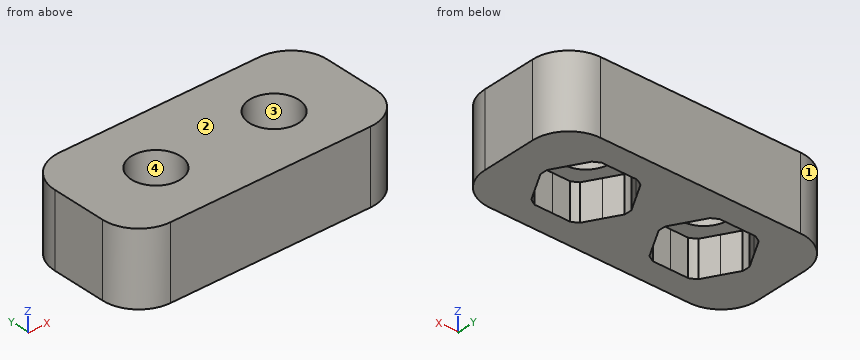
Solid Edge part; units mm, degrees
sketch "Sketch1" plane through (0, 0, 0) normal (0, 0, 1) x (1, 0, 0)
  line L0 (-4.5, -7) -> (17.5, -7)
  arc A0 (17.5, -7) -> (21.5, -3) centre (17.5, -3) ccw
  line L1 (21.5, -3) -> (21.5, 3)
  arc A1 (21.5, 3) -> (17.5, 7) centre (17.5, 3) ccw
  line L2 (17.5, 7) -> (-4.5, 7)
  arc A2 (-4.5, 7) -> (-8.5, 3) centre (-4.5, 3) ccw
  line L3 (-8.5, 3) -> (-8.5, -3)
  arc A3 (-8.5, -3) -> (-4.5, -7) centre (-4.5, -3) ccw
extrude "Protrusion1" add sketch "Sketch1" along normal blind 8
sketch "Sketch2" plane through (0, 0, 0) normal (0, 0, 1) x (1, 0, 0)
  line L0 (-1.9421, -4.225) -> (0, -4.225)
  line L1 (1.9421, -4.225) -> (0, -4.225)
  arc A0 (2.6879, -3.7944) -> (1.9421, -4.225) centre (0, 0) cw
  line L2 (2.6879, -3.7944) -> (3.659, -2.1125)
  line L3 (4.63, -0.4306) -> (3.659, -2.1125)
  arc A1 (4.63, 0.4306) -> (4.63, -0.4306) centre (0, 0) cw
  line L4 (4.63, 0.4306) -> (3.659, 2.1125)
  line L5 (2.6879, 3.7944) -> (3.659, 2.1125)
  arc A2 (1.9421, 4.225) -> (2.6879, 3.7944) centre (0, 0) cw
  line L6 (1.9421, 4.225) -> (0, 4.225)
  line L7 (-1.9421, 4.225) -> (0, 4.225)
  arc A3 (-2.6879, 3.7944) -> (-1.9421, 4.225) centre (0, 0) cw
  line L8 (-2.6879, 3.7944) -> (-3.659, 2.1125)
  line L9 (-4.63, 0.4306) -> (-3.659, 2.1125)
  arc A4 (-4.63, -0.4306) -> (-4.63, 0.4306) centre (0, 0) cw
  line L10 (-4.63, -0.4306) -> (-3.659, -2.1125)
  line L11 (-2.6879, -3.7944) -> (-3.659, -2.1125)
  arc A5 (-1.9421, -4.225) -> (-2.6879, -3.7944) centre (0, 0) cw
  line L12 (11.0579, -4.225) -> (13, -4.225)
  line L13 (14.9421, -4.225) -> (13, -4.225)
  arc A6 (15.6879, -3.7944) -> (14.9421, -4.225) centre (13, 0) cw
  line L14 (15.6879, -3.7944) -> (16.659, -2.1125)
  line L15 (17.63, -0.4306) -> (16.659, -2.1125)
  arc A7 (17.63, 0.4306) -> (17.63, -0.4306) centre (13, 0) cw
  line L16 (17.63, 0.4306) -> (16.659, 2.1125)
  line L17 (15.6879, 3.7944) -> (16.659, 2.1125)
  arc A8 (14.9421, 4.225) -> (15.6879, 3.7944) centre (13, 0) cw
  line L18 (14.9421, 4.225) -> (13, 4.225)
  line L19 (11.0579, 4.225) -> (13, 4.225)
  arc A9 (10.3121, 3.7944) -> (11.0579, 4.225) centre (13, 0) cw
  line L20 (10.3121, 3.7944) -> (9.341, 2.1125)
  line L21 (8.37, 0.4306) -> (9.341, 2.1125)
  arc A10 (8.37, -0.4306) -> (8.37, 0.4306) centre (13, 0) cw
  line L22 (8.37, -0.4306) -> (9.341, -2.1125)
  line L23 (10.3121, -3.7944) -> (9.341, -2.1125)
  arc A11 (11.0579, -4.225) -> (10.3121, -3.7944) centre (13, 0) cw
extrude "ExtrudedCutout_1" cut sketch "Sketch2" along normal blind 4
sketch "Sketch3" plane through (0, 0, 0) normal (0, 0, 1) x (1, 0, 0)
  circle A0 centre (0, 0) radius 2.7
  circle A1 centre (13, 0) radius 2.7
extrude "Cutout1" cut sketch "Sketch3" along normal through all
chamfer "Chamfer_1" [suppressed]
properties material "ABS Plastic, medium impact"
Input: part model. Units: mm. Frame: model coordinates. Face numbers are marked on the shaded views. Coordinates: 2 decimals unless noted, no trailing zeros. Loops run counter-clockwise (first coordinate to the right, second up) from the corner with the lowest first, then second, coordinate; pieces in that order, holes last. Notation, with made-up numbers: M 48,58 L 89,58 A33 ccw 89,87 Z; hole C 54,-2 d7. An arc over 180 degrees is marked long. Answer in a Markdown table with one row per item.
1. First-contact query: pin 1 (1 mm diameter, centred on x = 13.5, y = -1, fed in from +Z); pin 2 (1 mm diameter, centred on x = 15.5, y = 2.5, fed in from -Z). Flat tips, straight axial feed; report the tip coordinate or a pass-through.
Response:
| item | result |
|---|---|
| pin 1 | passes through |
| pin 2 | stops at z = 4 |
2. Material intervals for line 1 (X direction, y = 0, z = 4.95); line 2 (X direction, y = 0.25, z = 0.5); line 3 (Y direction, x = 0, z = 6.8), sorted ascending.
Response:
| item | result |
|---|---|
| line 1 | x = -8.5 to -2.7, 2.7 to 10.3, 15.7 to 21.5 |
| line 2 | x = -8.5 to -4.64, 4.64 to 8.36, 17.64 to 21.5 |
| line 3 | y = -7 to -2.7, 2.7 to 7 |
3. Section A-A, the plane y = 0. Output: boundary loops of the cut face in (x, z).
Response:
| item | result |
|---|---|
| outline | M -8.5,0 L -4.65,0 L -4.65,4 L -2.7,4 L -2.7,8 L -8.5,8 Z; M 2.7,4 L 4.65,4 L 4.65,0 L 8.35,0 L 8.35,4 L 10.3,4 L 10.3,8 L 2.7,8 Z; M 15.7,4 L 17.65,4 L 17.65,0 L 21.5,0 L 21.5,8 L 15.7,8 Z |
4. Section B-B, the plane z = 6. Output: boundary loops of the cut face in (x, y).
Response:
| item | result |
|---|---|
| outline | M -8.5,-3 A4 ccw -4.5,-7 L 17.5,-7 A4 ccw 21.5,-3 L 21.5,3 A4 ccw 17.5,7 L -4.5,7 A4 ccw -8.5,3 Z; hole C 0,0 d5.4; hole C 13,0 d5.4 |
5. Section C-C, the plane x = 4.25. Output: boundary loops of the cut face in (y, z), then the cut area to 3 significant figures.
Response:
| item | result |
|---|---|
| outline | M -7,0 L -1.09,0 L -1.09,4 L 1.09,4 L 1.09,0 L 7,0 L 7,8 L -7,8 Z |
| area | 103 mm2 |
6. Section D-D, the plane y = 6. Output: boundary loops of the cut face in (x, z).
Response:
| item | result |
|---|---|
| outline | M -7.15,0 L 20.15,0 L 20.15,8 L -7.15,8 Z |
7. Draft query along X for the marked faces 1, 2, 3 and 4. Return one class per face: pulls with the +X half, pulls with the -X half, needs draft (parallel to the pull), parting line crosses it, or undercut.
Response:
| item | result |
|---|---|
| face 1 | pulls with the -X half |
| face 2 | needs draft |
| face 3 | undercut |
| face 4 | undercut |
